For this review, take the finished solid that the model builds, in its own axes (mm). A direction names the side the tool comes from. Coordinates: 2 decimals unless noted, no trailing zeros. Loops run counter-clockwise (first coordinate to the right, second up) from the corner with the lowest first, then second, coordinate; pieces in that order, holes last. Notation, with made-up numbers: M 28,87.25 L 33,87.25 A17 cw 33,108.25 Z; hole C 2.25,20.5 d11. An arc over 180 degrees is marked long. Write item = value, one per line.
from build123d import *

# Parameters (mm, degrees)
F1_DEPTH = 12.986
F3_DEPTH = 3.89
F4_R     = 0.4


with BuildPart() as f1:
    # F0 (on Front) → F1 (new body)
    with BuildSketch(Plane.XZ):
        with BuildLine():
            Line((9.514224, 6.946266), (-9.445541, 6.946266))
            ThreePointArc((-9.445541, 6.946266), (-9.999012, 6.717011), (-10.228267, 6.16354))
            Line((-10.228267, 6.16354), (-10.228267, -6.159592))
            ThreePointArc((-10.228267, -6.159592), (-9.999012, -6.713063), (-9.445541, -6.942318))
            Line((-9.445541, -6.942318), (9.376897, -6.942318))
            ThreePointArc((9.376897, -6.942318), (9.927276, -6.716138), (10.159575, -6.168314))
            Line((10.159575, -6.168314), (10.296901, 6.154818))
            ThreePointArc((10.296901, 6.154818), (10.07077, 6.713918), (9.514224, 6.946266))
        make_face()
    extrude(amount=F1_DEPTH)

    # F2 (on face) → F3 (join)
    with BuildSketch(Plane(origin=(0, 0, 0), x_dir=(-1, 0, 0), z_dir=(0, 1, 0))):
        with BuildLine():
            Line((11.117267, -6.159592), (11.117267, 6.16354))
            ThreePointArc((11.117267, 6.16354), (10.62763, 7.345628), (9.445541, 7.835266))
            Line((9.445541, 7.835266), (-9.514224, 7.835266))
            ThreePointArc((-9.514224, 7.835266), (-10.70288, 7.339024), (-11.185846, 6.144911))
            Line((-11.185846, 6.144911), (-11.048519, -6.17822))
            ThreePointArc((-11.048519, -6.17822), (-10.552381, -7.348248), (-9.376897, -7.831318))
            Line((-9.376897, -7.831318), (9.445541, -7.831318))
            ThreePointArc((9.445541, -7.831318), (10.62763, -7.341681), (11.117267, -6.159592))
        make_face()
        with BuildLine():
            Line((-10.159575, -6.168314), (-10.296901, 6.154818))
            ThreePointArc((-10.296901, 6.154818), (-10.07077, 6.713918), (-9.514224, 6.946266))
            Line((-9.514224, 6.946266), (9.445541, 6.946266))
            ThreePointArc((9.445541, 6.946266), (9.999012, 6.717011), (10.228267, 6.16354))
            Line((10.228267, 6.16354), (10.228267, -6.159592))
            ThreePointArc((10.228267, -6.159592), (9.999012, -6.713063), (9.445541, -6.942318))
            Line((9.445541, -6.942318), (-9.376897, -6.942318))
            ThreePointArc((-9.376897, -6.942318), (-9.927276, -6.716138), (-10.159575, -6.168314))
        make_face(mode=Mode.SUBTRACT)
        with BuildLine():
            ThreePointArc((-9.514224, 6.946266), (-10.07077, 6.713918), (-10.296901, 6.154818))
            Line((-10.296901, 6.154818), (-10.159575, -6.168314))
            ThreePointArc((-10.159575, -6.168314), (-9.927276, -6.716138), (-9.376897, -6.942318))
            Line((-9.376897, -6.942318), (9.445541, -6.942318))
            ThreePointArc((9.445541, -6.942318), (9.999012, -6.713063), (10.228267, -6.159592))
            Line((10.228267, -6.159592), (10.228267, 6.16354))
            ThreePointArc((10.228267, 6.16354), (9.999012, 6.717011), (9.445541, 6.946266))
            Line((9.445541, 6.946266), (-9.514224, 6.946266))
        make_face()
    extrude(amount=F3_DEPTH)

    # F4
    f4_edges = [f1.edges().sort_by_distance(p)[0] for p in [
        (10.07077, -12.986, 6.713918),
        (0.034341, -12.986, 6.946266),
        (-9.999012, -12.986, 6.717011),
        (-10.228267, -12.986, 0.001974),
        (-9.999012, -12.986, -6.713063),
        (-0.034322, -12.986, -6.942318),
        (9.927276, -12.986, -6.716138),
        (10.228238, -12.986, -0.006748),
    ]]
    fillet(f4_edges, radius=F4_R)


solid = f1.part
Q1. For line 1 along Z through (x, y) = (-1, -0.25); line 2 along X through (y, z) = (-5, -6); line 3 along X through (y, z) = (0.25, 5), list the stretches that pass through material, from the lowest coordinate up.
Solved:
line_1 = -6.94 to 6.95
line_2 = -10.23 to 10.16
line_3 = -11.12 to 11.17
Q2. Add section A-A (x = 0.5). Write out the cut boundary in (y, z), and give its area (3 significant figures).
Solved:
outline = M -12.99,-6.54 A0.4 ccw -12.59,-6.94 L 0,-6.94 L 0,-7.83 L 3.89,-7.83 L 3.89,7.84 L 0,7.84 L 0,6.95 L -12.59,6.95 A0.4 ccw -12.99,6.55 Z
area = 241 mm²
Q3. Machinability: for faces 1 (the face through (-0.7, 0, 7.6)), 2 (the face through (0, -6, -6.942)), 3 (the face through (0, -6, 6.946)), 4 (the face through (-10.228, -6, 0)), which of the approach directions +Z, -Z, +X, -X, +Y, -Y give a long, thin tool a straight path to every point of the face, cutting with its end or side? Answer none if there is none.
Solved:
face_1 = -Y
face_2 = -Z, +X, -X, -Y
face_3 = +Z, +X, -X, -Y
face_4 = +Z, -Z, -X, -Y
Q4. For pin 1 Ø3 at (y, z) = (-3.5, -1) entering from -X; pin 2 Ø2 at (x, y) = (-2.5, -4) entering from -Z; pin 3 Ø6.5 at (x, y) = (-2.5, -6.5) entering from +Z, all flat-tipped, find the tip position at first contact; note any pin that passes through.
Solved:
pin_1 = -10.23
pin_2 = -6.94
pin_3 = 6.95
Q5. Add section B-B (y = -11.25). Write out the cut boundary in (x, z), and give its area (3 significant figures).
Solved:
outline = M -10.23,-6.16 A0.78 ccw -9.45,-6.94 L 9.38,-6.94 A0.78 ccw 10.16,-6.17 L 10.3,6.15 A0.78 ccw 9.51,6.95 L -9.45,6.95 A0.78 ccw -10.23,6.16 Z
area = 284 mm²
